Input: part model. Units: mm. Frame: model coordinates. Face numbers are marked on the shaded views. A direction names the side the tool comes from. Give positions to 0.01 mm unless a question says otherwise; leave off trailing zeros. Loops run counter-clockwise (first coordinate to the right, second up) from the corner with the lowest first, then second, coordinate; pieces in that order, holes last.
from build123d import *

# Parameters (mm, degrees)
RESSALTO_EXTRUS_O1_DEPTH = 80
ESBO_O2_W                = 40
ESBO_O2_H                = 33
ESBO_O2_W_2              = 25.6
CORTE_EXTRUS_O1_DEPTH    = 12
ESBO_O4_R                = 2
CORTE_EXTRUS_O3_DEPTH    = 12
ESBO_O6_W                = 10
ESBO_O6_H                = 20
RESSALTO_EXTRUS_O2_DEPTH = 10
ESBO_O7_R                = 1.75
CORTE_EXTRUS_O4_DEPTH    = 15
CORTE_EXTRUS_O5_DEPTH    = 5
ESBO_O10_R               = 5
ESBO_O10_R_2             = 2.75
RESSALTO_EXTRUS_O3_DEPTH = 5
ESBO_O11_W               = 20
ESBO_O11_H               = 20
ESBO_O11_W_2             = 25
ESBO_O11_H_2             = 10
CORTE_EXTRUS_O7_DEPTH    = 60
ESBO_O13_W               = 30
ESBO_O13_H               = 47
CORTE_EXTRUS_O9_DEPTH    = 168
FILETE1_R                = 1.5
ESBO_O14_R               = 1.75
CORTE_EXTRUS_O10_DEPTH   = 14.5
CORTE_EXTRUS_O11_DEPTH   = 2.5
FILETE2_R                = 1


with BuildPart() as part:
    # Esboço1 → Ressalto-extrusão1 (new body)
    with BuildSketch(Plane.XY):
        Polygon((-2.5, 45), (-15, 45), (-15, 2), (-10, 2), (-10, 35), (10, 35), (10, -35), (-15, -35), (-15, -45), (15, -45), (15, 45), (2.5, 45), (5, 40), (-5, 40), align=None)
    extrude(amount=RESSALTO_EXTRUS_O1_DEPTH)

    # Esboço2 → Corte-extrusão1 (cut)
    with BuildSketch(Plane.ZY.offset(15)):
        with Locations((27.2, 18.5)):
            Rectangle(ESBO_O2_W, ESBO_O2_H)
        with Locations((67.2, 18.5)):
            Rectangle(ESBO_O2_W_2, ESBO_O2_H)
    extrude(amount=-CORTE_EXTRUS_O1_DEPTH, mode=Mode.SUBTRACT)

    # Esboço4 → Corte-extrusão3 (cut)
    with BuildSketch(Plane(origin=(-10, 0, 0), x_dir=(0, 0, -1), z_dir=(1, 0, 0))):
        with Locations(Location((-3.104223841, 17.002484575, 0), (0, 0, 90))):
            Circle(ESBO_O4_R)
        with Locations(Location((-3.104223841, 7.000828192, 0), (0, 0, 90))):
            Circle(ESBO_O4_R)
        with Locations(Location((-51.210481376, 17.002484575, 0), (0, 0, 90))):
            Circle(ESBO_O4_R)
        with Locations(Location((-51.210481376, 7.000828192, 0), (0, 0, 90))):
            Circle(ESBO_O4_R)
    extrude(amount=-CORTE_EXTRUS_O3_DEPTH, mode=Mode.SUBTRACT)

    # Esboço6 → Ressalto-extrusão2 (add)
    with BuildSketch(Plane.ZY.offset(15)):
        with Locations((85, 25)):
            Rectangle(ESBO_O6_W, ESBO_O6_H)
        Polygon((80, 35), (90, 35), (80, 45), align=None)
    extrude(amount=-RESSALTO_EXTRUS_O2_DEPTH)

    # Esboço7 → Corte-extrusão4 (cut)
    with BuildSketch(Plane.ZY.offset(15)):
        with Locations(Location((85, 20, 0), (0, 0, 270))):
            Circle(ESBO_O7_R)
    extrude(amount=-CORTE_EXTRUS_O4_DEPTH, mode=Mode.SUBTRACT)

    # Esboço8 → Corte-extrusão5 (cut)
    with BuildSketch(Plane.ZY.offset(15)):
        Polygon((85, 23.75277675), (81.75, 21.876388375), (81.75, 18.123611625), (85, 16.24722325), (88.25, 18.123611625), (88.25, 21.876388375), align=None)
    extrude(amount=-CORTE_EXTRUS_O5_DEPTH, mode=Mode.SUBTRACT)

    # Esboço10 → Ressalto-extrusão3 (add)
    # profile 1 of 3: a face of its own
    with BuildSketch(Plane(origin=(15, 0, 0), x_dir=(0, 0, -1), z_dir=(1, 0, 0))):
        with BuildLine():
            Line((-80, 25), (-85, 25))
            ThreePointArc((-85, 25), (-81.464466094, 23.535533906), (-80, 20))
            Line((-80, 20), (-80, 25))
        make_face()
    # profile 2 of 3: a face of its own
    with BuildSketch(Plane(origin=(15, 0, 0), x_dir=(0, 0, -1), z_dir=(1, 0, 0))):
        with Locations((-85, 20)):
            Circle(ESBO_O10_R)
        with Locations(Location((-85, 20, 0), (0, 0, 90))):
            Circle(ESBO_O10_R_2, mode=Mode.SUBTRACT)
    # profile 3 of 3: a face of its own
    with BuildSketch(Plane(origin=(15, 0, 0), x_dir=(0, 0, -1), z_dir=(1, 0, 0))):
        with BuildLine():
            Line((-80, 15), (-80, 20))
            ThreePointArc((-80, 20), (-81.464466094, 16.464466094), (-85, 15))
            Line((-85, 15), (-80, 15))
        make_face()
    extrude(amount=-RESSALTO_EXTRUS_O3_DEPTH)

    # Esboço11 → Corte-extrusão7 (cut)
    with BuildSketch(Plane.XY.offset(80)):
        with Locations((5, 35)):
            Rectangle(ESBO_O11_W, ESBO_O11_H)
        Polygon((10, -45), (15, -45), (15, 15), (10, 15), (10, -35), align=None)
        with Locations((-2.5, -40)):
            Rectangle(ESBO_O11_W_2, ESBO_O11_H_2)
    extrude(amount=-CORTE_EXTRUS_O7_DEPTH, mode=Mode.SUBTRACT)

    # Esboço13 → Corte-extrusão9 (cut)
    with BuildSketch(Plane.XY.offset(20)):
        with Locations((0, -21.5)):
            Rectangle(ESBO_O13_W, ESBO_O13_H)
    extrude(amount=-CORTE_EXTRUS_O9_DEPTH, mode=Mode.SUBTRACT)

    # Filete1
    filete1_edges = [part.edges().sort_by_distance(p)[0] for p in [
        (2.5, 45, 10),
        (-2.5, 45, 10),
    ]]
    fillet(filete1_edges, radius=FILETE1_R)

    # Esboço14 → Corte-extrusão10 (cut)
    with BuildSketch(Plane(origin=(0, 40, 0), x_dir=(1, 0, 0), z_dir=(0, 1, 0))):
        with Locations(Location((0, -10, 0), (0, 0, 270))):
            Circle(ESBO_O14_R)
    extrude(amount=-CORTE_EXTRUS_O10_DEPTH, mode=Mode.SUBTRACT)

    # Esboço15 → Corte-extrusão11 (cut)
    with BuildSketch(Plane.XZ.offset(-35)):
        Polygon((0, 13.75277675), (-3.25, 11.876388375), (-3.25, 8.123611625), (0, 6.24722325), (3.25, 8.123611625), (3.25, 11.876388375), align=None)
    extrude(amount=-CORTE_EXTRUS_O11_DEPTH, mode=Mode.SUBTRACT)

    # Filete2
    filete2_edges = [part.edges().sort_by_distance(p)[0] for p in [
        (-5, 40, 10),
        (5, 40, 10),
    ]]
    fillet(filete2_edges, radius=FILETE2_R)


solid = part.part
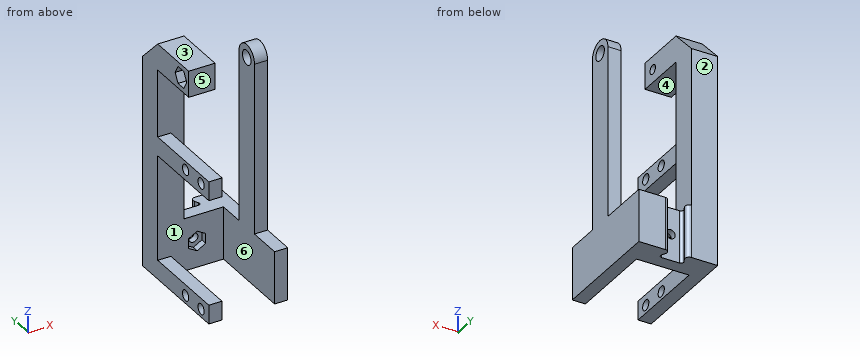
(1) Cut plane A-A (x = 12.5). Return the cut outline in (y, z).
Values follow:
outline: (2, 0) - (45, 0) - (45, 20) - (25, 20) - (25, 85) arc R5 ccw to (15, 85) - (15, 20) - (2, 20) - close; hole circle Ø5.5 at (20, 85)
(2) Pin query (flat end, axial travel): pin 1 Ø5.5 at (x, y) = (13, 11.5) entering from +Z; pin 2 Ø2 at (x, z) = (-4.5, 65.5) entering from +Y; pin 3 Ø6 at (y, z) = (9.5, 65) entering from +X; pin 4 Ø6 at (x, z) = (-5, 48.5) entering from -Y. Return the tip coordinate at first contact, or that it passes through.
Values follow:
pin 1: stops at z = 20
pin 2: stops at y = 45
pin 3: passes through
pin 4: stops at y = 35
(3) Cut plane D-D (y = 20). Return the cut outline in (x, z), and give its area (4 significant figures).
Values follow:
outline: (-15, 0) - (-10, 0) - (-10, 7.2) - (-15, 7.2) - close; (-15, 47.2) - (-10, 47.2) - (-10, 54.4) - (-15, 54.4) - close; (-15, 80) - (-5, 80) - (-5, 83.25) - (-10, 83.25) - (-10, 81.75) - (-15, 81.75) - close; (-15, 88.25) - (-10, 88.25) - (-10, 86.75) - (-5, 86.75) - (-5, 90) - (-15, 90) - close; (10, 0) - (15, 0) - (15, 82.25) - (10, 82.25) - close; (10, 87.75) - (15, 87.75) - (15, 90) - (10, 90) - close
area: 544.5 mm2
(4) Mould query, pull axis Z, two halves, no side actions, for the marked faces 1, 2 and 3. Classes: +Z half, -Z half, draft (parallel to the pull), parting line (faces both ways), or undercut.
Values follow:
face 1: undercut
face 2: draft
face 3: +Z half
(5) Cut plane B-B (y = 27). Return the cut outline in (x, z), and give its area (3 significant figures).
Values follow:
outline: (-15, 0) - (-10, 0) - (-10, 7.2) - (-15, 7.2) - close; (-15, 47.2) - (-10, 47.2) - (-10, 54.4) - (-15, 54.4) - close; (-15, 80) - (-5, 80) - (-5, 90) - (-15, 90) - close; (10, 0) - (15, 0) - (15, 20) - (10, 20) - close
area: 272 mm2
(6) Ray query, probe 1 along X at (y, z) = (19.5, 54); probe 2 along Y at (x, z) = (-7.2, 85); probe 3 along Z at (x, y) = (12.15, 20). Return the intervals inside material, ascending.
Values follow:
probe 1: x = -15 to -10, 10 to 15
probe 2: y = 15 to 18.25, 21.75 to 40
probe 3: z = 0 to 82.25, 87.75 to 90
(7) Cut plane C-C (z = 30). Return the cut outline in (x, y).
Values follow:
outline: (-15, 35) - (-5, 35) - (-5, 45) - (-15, 45) - close; (10, 15) - (15, 15) - (15, 25) - (10, 25) - close
(8) Reachability of the marked faces 4, 5 and 6 from +Z, -Z, +X, -X, +Y, -Y: full face, straight path, thin tool, end or side. Return the list, or none.
Values follow:
face 4: -X, -Y
face 5: +Z, +X, -X, -Y
face 6: +Z, -Z, -Y
